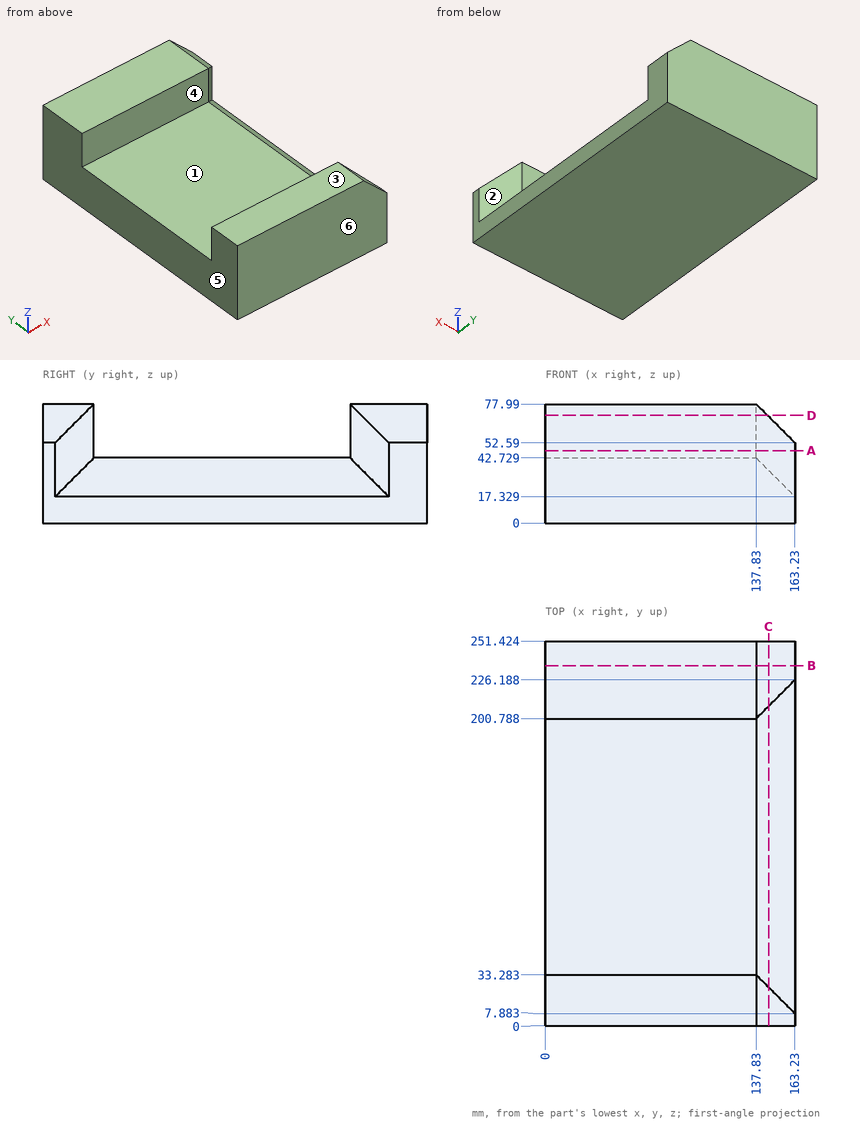
Verification items for this drawing (mm, ordinates from the low corner). A direction names the side the tool comes from. Coordinates: 2 decimals unless noted, no trailing zeros. Order: outer loops, then holes, each group sorted by start corner. A loop starts at its lowest first (then second) coordinate and runs counter-clockwise, first axis right, second up. Notation, with made-up numbers: (31.25, 39.25) - (79.25, 39.25) arc R27 cw to (79.25, 57.25) - close; hole circle Ø1 at (-13, -2.5). An arc over 180 degrees is marked (long way). Answer in a Markdown table with one row per item. Add a question column.
1. Section check C-C (x = 146). Enter the section's corners in (y, z) (1 decimal), plus the area to 3 significant figures.
2. Section check A-A (z = 47.5). Enter the section's corners in (x, y) (1 decimal), plus the area to 3 significant figures.
3. Draft check along Y on the marked faces 4, 5 and 6. Enter one of: +Y half, -Y half, draft (parallel to the pull), parting line (faces both ways), or undercut.
4. Section check D-D (z = 70.5). Enter the section's corners in (x, y) (1 decimal).
5. Section check B-B (y = 235.5). Enter the section's corners in (x, z).
6. Material ranges on L1, parallel to Y at x = 88.5, z = 68.5 (1 decimal); L2, parallel to Z at x = 81, y = 111; L3, parallel to X at y = 120.5, z = 35, recorded low to high. Write a range as [from, to].
7. Gauge pin test, flat end, axial feed: pin 1 Ø4 at (y, z) = (97.5, 28) entering from +X. Record the tip position at first contact, or that the pin passes through.
8. Access from +Z, -Z, +X, -X, +Y, -Y to the whole of each face (thin tool, end or side, straight path). Record for the marked faces 1, 2 and 3.
Data:
| question | item | result |
|---|---|---|
| 1 | outline | (0, 0) - (251.4, 0) - (251.4, 69.8) - (209, 69.8) - (209, 34.6) - (25.1, 34.6) - (25.1, 69.8) - (0, 69.8) - close |
| 1 | area | 11,100 mm² |
| 2 | outline | (0, 0) - (163.2, 0) - (163.2, 7.9) - (137.8, 33.3) - (0, 33.3) - close; (0, 200.8) - (137.8, 200.8) - (163.2, 226.2) - (163.2, 251.4) - (0, 251.4) - close |
| 2 | area | 13,100 mm² |
| 3 | face 4 | undercut |
| 3 | face 5 | draft |
| 3 | face 6 | -Y half |
| 4 | outline | (0, 0) - (145.3, 0) - (145.3, 25.8) - (137.8, 33.3) - (0, 33.3) - close; (0, 200.8) - (137.8, 200.8) - (145.3, 208.3) - (145.3, 251.4) - (0, 251.4) - close |
| 5 | outline | (0, 0) - (163.23, 0) - (163.23, 52.59) - (137.83, 77.99) - (0, 77.99) - close |
| 6 | L1 | y = [0, 33.3], [200.8, 251.4] |
| 6 | L2 | z = [0, 42.73] |
| 6 | L3 | x = [0, 145.56] |
| 7 | pin 1 | stops at x = 154.56 |
| 8 | face 1 | +Z, +X, -X |
| 8 | face 2 | +Z, +X |
| 8 | face 3 | +Z, +X, -X, +Y, -Y |
